```python
from build123d import *

# Parameters (mm, degrees)
BOSS_EXTRUDE1_DEPTH           = 0.79375
BOSS_EXTRUDE1_TAPER           = 30
SKETCH3_R                     = 0.79375
BOSS_EXTRUDE2_DEPTH           = 0.254
BOSS_EXTRUDE2_DRAFT           = 30
BOSS_EXTRUDE2_PROFILE_2_DEPTH = 0.254
BOSS_EXTRUDE2_PROFILE_2_DRAFT = 30
BOSS_EXTRUDE2_PROFILE_3_DEPTH = 0.254
BOSS_EXTRUDE2_PROFILE_3_DRAFT = 30
BOSS_EXTRUDE2_PROFILE_4_DEPTH = 0.254
BOSS_EXTRUDE2_PROFILE_4_DRAFT = 30
FILLET1_R                     = 0.381


with BuildPart() as part:
    # Sketch2 → Boss-Extrude1 (new body)
    with BuildSketch(Plane(origin=(0, 15.875, 0), x_dir=(1, 0, 0), z_dir=(0, 1, 0))):
        Polygon((-169.8625, 42.8625), (-169.8625, 17.4625), (-163.5125, 17.4625), (-163.5125, 26.9875), (-144.4625, 26.9875), (-144.4625, 33.3375), (-163.5125, 33.3375), (-163.5125, 42.8625), align=None)
    extrude(amount=BOSS_EXTRUDE1_DEPTH, taper=BOSS_EXTRUDE1_TAPER)


with BuildPart() as boss_extrude2_tool:
    # Sketch3 → Boss-Extrude2 (with draft: the straight prism first)
    with BuildSketch(Plane(origin=(0, 16.66875, 0), x_dir=(1, 0, 0), z_dir=(0, 1, 0))):
        with Locations((-147.6375, 30.1625)):
            Circle(SKETCH3_R)
    extrude(amount=BOSS_EXTRUDE2_DEPTH)
    # Boss-Extrude2: the draft: its side faces are tilted about the plane it starts from
    boss_extrude2_sides = [boss_extrude2_tool.faces().sort_by_distance(p)[0] for p in [
        (-148.43125, 16.79575, -30.1625),
    ]]
    draft(boss_extrude2_sides, Plane(origin=(0, 16.66875, 0), x_dir=(1, 0, 0), z_dir=(0, 1, 0)), BOSS_EXTRUDE2_DRAFT)


with BuildPart() as part_1:
    add(part.part)

    # Boss-Extrude2: add boss_extrude2_tool
    add(boss_extrude2_tool.part)


with BuildPart() as boss_extrude2_profile_2_tool:
    # Sketch3 → Boss-Extrude2 profile 2 (with draft: the straight prism first)
    with BuildSketch(Plane(origin=(0, 16.66875, 0), x_dir=(1, 0, 0), z_dir=(0, 1, 0))):
        with Locations((-160.3375, 30.1625)):
            Circle(SKETCH3_R)
    extrude(amount=BOSS_EXTRUDE2_PROFILE_2_DEPTH)
    # Boss-Extrude2 profile 2: the draft: its side faces are tilted about the plane it starts from
    boss_extrude2_profile_2_sides = [boss_extrude2_profile_2_tool.faces().sort_by_distance(p)[0] for p in [
        (-161.13125, 16.79575, -30.1625),
    ]]
    draft(boss_extrude2_profile_2_sides, Plane(origin=(0, 16.66875, 0), x_dir=(1, 0, 0), z_dir=(0, 1, 0)), BOSS_EXTRUDE2_PROFILE_2_DRAFT)


with BuildPart() as part_2:
    add(part_1.part)

    # Boss-Extrude2 profile 2: add boss_extrude2_profile_2_tool
    add(boss_extrude2_profile_2_tool.part)


with BuildPart() as boss_extrude2_profile_3_tool:
    # Sketch3 → Boss-Extrude2 profile 3 (with draft: the straight prism first)
    with BuildSketch(Plane(origin=(0, 16.66875, 0), x_dir=(1, 0, 0), z_dir=(0, 1, 0))):
        with Locations((-166.6875, 39.6875)):
            Circle(SKETCH3_R)
    extrude(amount=BOSS_EXTRUDE2_PROFILE_3_DEPTH)
    # Boss-Extrude2 profile 3: the draft: its side faces are tilted about the plane it starts from
    boss_extrude2_profile_3_sides = [boss_extrude2_profile_3_tool.faces().sort_by_distance(p)[0] for p in [
        (-167.48125, 16.79575, -39.6875),
    ]]
    draft(boss_extrude2_profile_3_sides, Plane(origin=(0, 16.66875, 0), x_dir=(1, 0, 0), z_dir=(0, 1, 0)), BOSS_EXTRUDE2_PROFILE_3_DRAFT)


with BuildPart() as part_3:
    add(part_2.part)

    # Boss-Extrude2 profile 3: add boss_extrude2_profile_3_tool
    add(boss_extrude2_profile_3_tool.part)


with BuildPart() as boss_extrude2_profile_4_tool:
    # Sketch3 → Boss-Extrude2 profile 4 (with draft: the straight prism first)
    with BuildSketch(Plane(origin=(0, 16.66875, 0), x_dir=(1, 0, 0), z_dir=(0, 1, 0))):
        with Locations((-166.6875, 20.6375)):
            Circle(SKETCH3_R)
    extrude(amount=BOSS_EXTRUDE2_PROFILE_4_DEPTH)
    # Boss-Extrude2 profile 4: the draft: its side faces are tilted about the plane it starts from
    boss_extrude2_profile_4_sides = [boss_extrude2_profile_4_tool.faces().sort_by_distance(p)[0] for p in [
        (-167.48125, 16.79575, -20.6375),
    ]]
    draft(boss_extrude2_profile_4_sides, Plane(origin=(0, 16.66875, 0), x_dir=(1, 0, 0), z_dir=(0, 1, 0)), BOSS_EXTRUDE2_PROFILE_4_DRAFT)


with BuildPart() as part_4:
    add(part_3.part)

    # Boss-Extrude2 profile 4: add boss_extrude2_profile_4_tool
    add(boss_extrude2_profile_4_tool.part)

    # Fillet1
    fillet1_edges = [part_4.edges().sort_by_distance(p)[0] for p in [
        (-148.284603032, 16.92275, -30.1625),
        (-160.984603032, 16.92275, -30.1625),
        (-167.334603032, 16.92275, -39.6875),
        (-167.334603032, 16.92275, -20.6375),
    ]]
    fillet(fillet1_edges, radius=FILLET1_R)


solid = part_4.part
```
The listing builds one solid part. Answer for the finished solid, in the listing's coordinates (mm). A direction names the side the tool comes from. Coordinates: 2 decimals unless noted, no trailing zeros. Use one line per item in the form item = value. Start each with the question number.
Item 1: A tool of negligible diameter and unlimited length cuts with its end or side. For faces 1 (the face through (-162, 16.669, -29)), 2 (the face through (-160.3, 16.923, -30.2)), from which of +Z, -Z, +X, -X, +Y, -Y can it reach the whole face along a straight path? Write none if from no direction.
Item 2: Flat-ended cylindrical pins translate along their axes: pin 1 Ø8 at (x, z) = (-166, -29.5) entering from +Y; pin 2 Ø6 at (x, z) = (-151.5, -23.5) entering from -Y. Find the tip coordinate at first contact, or state that the pin passes through.
Item 3: Consider L1, parallel to Y at x = -161.75, z = -32.75 (3 decimals); L2, parallel to Z at x = -167, y = 16.85; L3, parallel to Z at x = -164, y = 16.6. Determine where each line is inside the solid, lowest interval first. Write a range as [from, to].
Answer key:
q1.face_1 = +Y
q1.face_2 = +Z, -Z, +X, -X, +Y
q2.pin_1 = 16.67
q2.pin_2 = through
q3.L1 = [15.875, 16.669]
q3.L2 = [-40.26, -39.12], [-21.21, -20.07]
q3.L3 = [-42.44, -17.88]
